from build123d import *

# Parameters (mm, degrees)
BOSS_EXTRUDE1_DEPTH = 25.4
FILLET1_R           = 12.7
SKETCH4_R           = 3.175
CUT_EXTRUDE2_DEPTH  = 12.7


with BuildPart() as part:
    # Sketch1 → Boss-Extrude1 (new body)
    with BuildSketch(Plane(origin=(0, 0, 0), x_dir=(1, 0, 0), z_dir=(0, 1, 0))):
        with BuildLine():
            Line((-1.27, 50.8), (-1.27, 25.4))
            Line((-1.27, 25.4), (-0.253683094, 5.073661881))
            ThreePointArc((-0.253683094, 5.073661881), (0, 4.832346036), (0.253683094, 5.073661881))
            Line((0.253683094, 5.073661881), (1.27, 25.4))
            Line((1.27, 25.4), (1.27, 50.8))
            Line((1.27, 50.8), (0.253683094, 71.126338119))
            ThreePointArc((0.253683094, 71.126338119), (0, 71.367653964), (-0.253683094, 71.126338119))
            Line((-0.253683094, 71.126338119), (-1.27, 50.8))
        make_face()
    extrude(amount=BOSS_EXTRUDE1_DEPTH)

    # Fillet1
    # the kernel refuses this fillet: 12.7 mm, written as the material it takes off along each edge
    with BuildSketch(Plane(origin=(-1.27, -0.793254525, -25.4), x_dir=(0, 0, -1), z_dir=(0, 1, 0)), Plane(origin=(-1.27, -0.793254525, -50.8), x_dir=(0.04993761694389363, 0, -0.9987523388778445), z_dir=(0, 1, 0)), Plane(origin=(1.27, -0.793254525, -50.8), x_dir=(0, 0, 1), z_dir=(0, 1, 0)), Plane(origin=(1.27, -0.793254525, -25.4), x_dir=(-0.04993761694389503, 0, 0.9987523388778445), z_dir=(0, 1, 0))) as fillet1_piece_1:
        with BuildLine():
            CenterArc((FILLET1_R * 0.0249843945008, -FILLET1_R), FILLET1_R, 90, 2.862405226)
            Line((-FILLET1_R * 0.0249532224431, -FILLET1_R * 0.00124766112216), (0, 0))
            Line((0, 0), (FILLET1_R * 0.0249843945008, 0))
        make_face()
    extrude(amount=26.986509051, mode=Mode.SUBTRACT)

    # Sketch4 → Cut-Extrude2 (cut)
    with BuildSketch(Plane(origin=(0, 0, 0), x_dir=(1, 0, 0), z_dir=(0, 1, 0))):
        with Locations((0, 6.35)):
            Circle(SKETCH4_R)
    extrude(amount=CUT_EXTRUDE2_DEPTH, mode=Mode.SUBTRACT)


solid = part.part
Check sheet for the modelled part. Datum: model origin and axes. Units: mm. Give positions to 0.01 mm unless a question says otherwise; leave off trailing zeros. Loops run counter-clockwise (first coordinate to the right, second up) from the corner with the lowest first, then second, coordinate; pieces in that order, holes last. Notation, with made-up numbers: M -17.75,86 L 40.25,86 A26 ccw 40.25,124 Z; hole C 53.5,-26 d5. An arc over 180 degrees is marked long. Use a Markdown table: item, result. Add a question column.
Q1. Go/stop test with flat-tipped pins: pin 1 (1 mm diameter, centred on x = 0, z = -6, fed in from -Y); pin 2 (4 mm diameter, centred on y = 7.5, z = -14.5, fed in from +X) (3 decimals); pin 3 (5 mm diameter, centred on y = 18.5, z = -61, fed in from +X) (3 decimals). Record where each tip stops, or that it passes through.
Q2. Sectioned sample at A-A, the plane y = 20. Record the cut outline in (x, z).
Q3. Scan lines: line 1 along Z through (x, y) = (0.05, 3); line 2 along X through (y, z) = (18.75, -59); line 3 along X through (y, z) = (14, -20). Record each from-to range of solid material in increasing order. Write a range as [from, to].
Q4. Sectioned sample at B-B, the plane y = 8.5. Record the cut outline in (x, z) (3 decimals), then the cut area to 3 significant figures.
Verdict:
| question | item | result |
|---|---|---|
| 1 | pin 1 | y = 12.7 |
| 1 | pin 2 | x = 0.825 |
| 1 | pin 3 | x = 0.885 |
| 2 | outline | M -1.27,-50.48 A12.7 ccw -1.25,-51.12 L -0.25,-71.13 A0.25 ccw 0.25,-71.13 L 1.25,-51.12 A12.7 ccw 1.27,-50.48 L 1.27,-25.72 A12.7 ccw 1.25,-25.08 L 0.25,-5.07 A0.25 ccw -0.25,-5.07 L -1.25,-25.08 A12.7 ccw -1.27,-25.72 Z |
| 3 | line 1 | [-71.36, -9.52] |
| 3 | line 2 | [-0.86, 0.86] |
| 3 | line 3 | [-1, 1] |
| 4 | outline | M -1.27,-50.483 A12.7 ccw -1.254,-51.117 L -0.254,-71.126 A0.254 ccw 0.254,-71.126 L 1.254,-51.117 A12.7 ccw 1.27,-50.483 L 1.27,-25.717 A12.7 ccw 1.254,-25.083 L 0.474,-9.489 A3.175 cw -0.474,-9.489 L -1.254,-25.083 A12.7 ccw -1.27,-25.717 Z |
| 4 | area | 123 mm^2 |
